For this review, use the dimensioned drawing (mm, ordinates from the lowest corner) and the shaded views. A direction names the side the tool comes from. Give positions to 0.01 mm unless a question says otherwise; leave off trailing zeros. Order: outer loops, then holes, each group sorted by start corner. A loop starts at its lowest first (then second) coordinate and runs counter-clockwise, first axis right, second up. Notation, with made-up numbers: (-12, -6) - (30, -6) arc R10 ccw to (30, 3) - close; hole circle Ø10 at (12.5, 63). An arc over 180 degrees is marked (long way). Use a Markdown table: item, result. Add a question column.
1) We need section B-B on x = 12.5. Write out the cut boundary in (y, z), then the cut area to 3 significant figures.
2) Wall thickness on L1, parallel to Z at x = 142.5, y = 0.6; L2, parallel to X at y = 0.7, z = 132.5; L3, parallel to Z at x = 33.5, y = 20: over which ranges is each line inside the solid? List them lowest first.
3) We need section C-C on z = 132.5. Write out the cut boundary in (x, y), then the cut area to 3 significant figures.
4) We need section D-D on z = 90. Write out the cut boundary in (x, y), then the cut area to 3 significant figures.
5) Clearance check with flat-ended pins moving along their axes: P1, Ø6, axis at x = 16.5, z = 21, coming from the +Y side; P2, Ø12, axis at y = 115, z = 62, coming from the +X side; P3, Ø6, axis at x = 44, z = 127.5, coming from the -Y side; P4, Ø2, axis at y = 44, z = 53.5, coming from the -X side. State where each tip first meets the part, or that it passes through.
6) We need section A-A on y = 39. Give the number of separate pieces and of enclosed holes in the cut face, then the cut area to 3 significant figures.
7) Mouldability with a two-part tool opening along Z and no side actions: class the marked faces 5, 6 and 7 as released by +Z, released by -Z, zero draft, split by the parting line, or undercut.
8) Machinability: for the marked faces 1, 2, 3 and 4, which of the approach directions +Z, -Z, +X, -X, +Y, -Y give a long, thin tool a straight path to every point of the face, cutting with its end or side? Answer none if there is none.
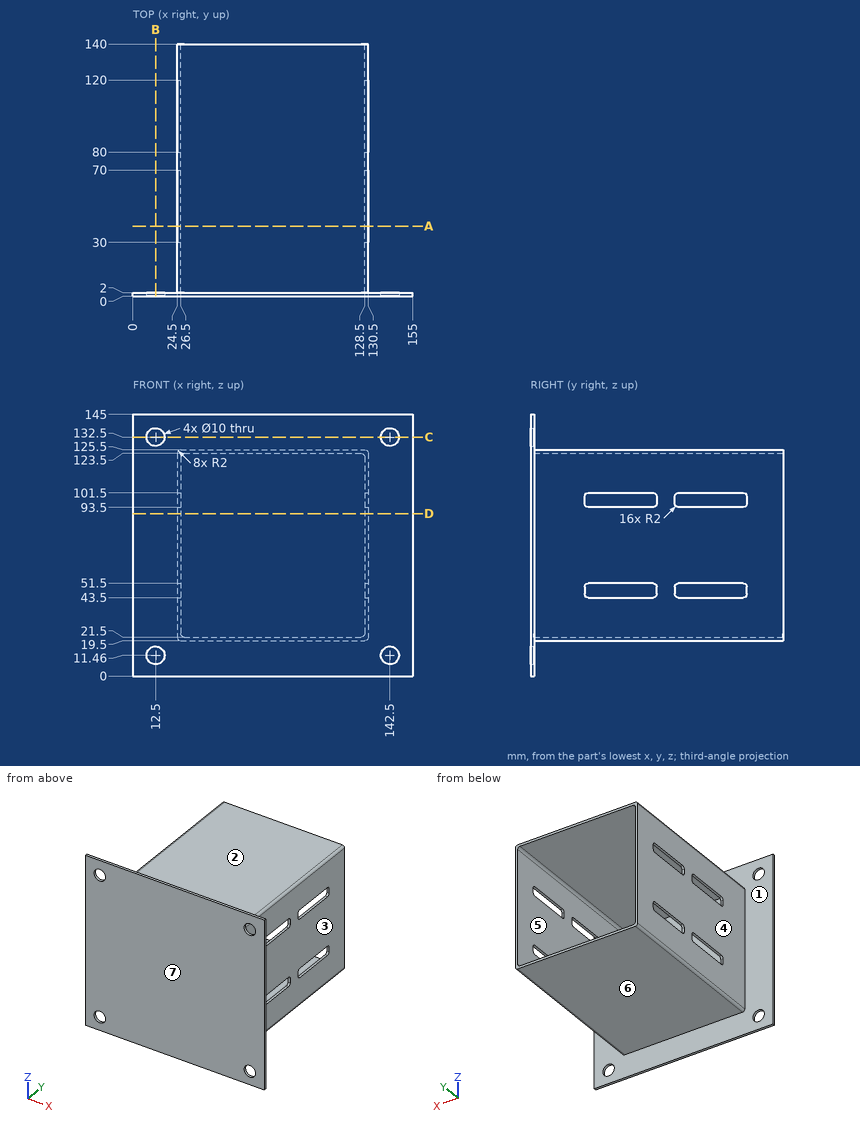
Checked values:
| question | item | result |
|---|---|---|
| 1 | outline | (0, 0) - (2, 0) - (2, 6.46) - (0, 6.46) - close; (0, 16.46) - (2, 16.46) - (2, 127.5) - (0, 127.5) - close; (0, 137.5) - (2, 137.5) - (2, 145) - (0, 145) - close |
| 1 | area | 250 mm² |
| 2 | L1 | 0 to 6.46, 16.46 to 127.5, 137.5 to 145 |
| 2 | L2 | 0 to 7.5, 17.5 to 137.5, 147.5 to 155 |
| 2 | L3 | 19.5 to 21.5, 123.5 to 125.5 |
| 3 | outline | (0, 0) - (7.5, 0) - (7.5, 2) - (0, 2) - close; (17.5, 0) - (137.5, 0) - (137.5, 2) - (17.5, 2) - close; (147.5, 0) - (155, 0) - (155, 2) - (147.5, 2) - close |
| 3 | area | 270 mm² |
| 4 | outline | (0, 0) - (155, 0) - (155, 2) - (130.5, 2) - (130.5, 140) - (128.5, 140) - (128.5, 2) - (26.5, 2) - (26.5, 140) - (24.5, 140) - (24.5, 2) - (0, 2) - close |
| 4 | area | 862 mm² |
| 5 | P1 | y = 2 |
| 5 | P2 | x = 130.5 |
| 5 | P3 | y = 0 |
| 5 | P4 | x = 24.5 |
| 6 | separate pieces | 4 |
| 6 | enclosed holes | 0 |
| 6 | area | 768 mm² |
| 7 | face 5 | undercut |
| 7 | face 6 | released by -Z |
| 7 | face 7 | zero draft |
| 8 | face 1 | +Y |
| 8 | face 2 | +Z, +X, -X, +Y |
| 8 | face 3 | +Z, -Z, +X, +Y |
| 8 | face 4 | +Z, -Z, -X, +Y |
